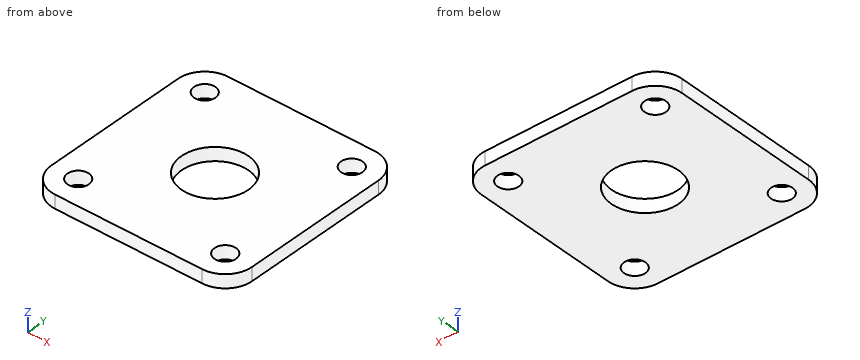
```python
from build123d import *

# Parameters (mm, degrees)
CYLINDER057_R       = 5
CYLINDER057_DEPTH   = 15
CYLINDER058_R       = 1.6
CYLINDER058_DEPTH   = 20
ARRAY001029_X_COUNT = 2
ARRAY001029_X_PITCH = 22
ARRAY001029_Y_COUNT = 2
ARRAY001029_Y_PITCH = 22
BOX007_W            = 30
BOX007_H            = 30
BOX007_DEPTH        = 2
FILLET013_R         = 4


with BuildPart() as side_bearing_central_hole_cylinder001:
    # Cylinder057 → Cylinder057 (new body)
    with BuildSketch(Plane(origin=(15, 15, -4), x_dir=(1, 0, 0), z_dir=(0, 0, 1))):
        Circle(CYLINDER057_R)
    extrude(amount=CYLINDER057_DEPTH)


with BuildPart() as fusion039:
    # Cylinder058 → Cylinder058 (new body)
    with BuildSketch(Plane(origin=(4, 4, -7), x_dir=(1, 0, 0), z_dir=(0, 0, 1))):
        Circle(CYLINDER058_R)
    extrude(amount=CYLINDER058_DEPTH)

    # Array001029 X: Fusion039 ×2


with BuildPart() as fusion039_1:
    add(fusion039.part)
    with Locations(*[(i * ARRAY001029_X_PITCH, 0, 0) for i in range(1, ARRAY001029_X_COUNT)]):
        add(fusion039.part)

    # Array001029 Y: Fusion039 ×2


with BuildPart() as fusion039_2:
    add(fusion039_1.part)
    with Locations(*[(0, i * ARRAY001029_Y_PITCH, 0) for i in range(1, ARRAY001029_Y_COUNT)]):
        add(fusion039_1.part)

    # Fusion039: union side bearing central hole cylinder001
    add(side_bearing_central_hole_cylinder001.part)


with BuildPart() as bearing_cover_fillet:
    # Box007 → Box007 (new body)
    with BuildSketch(Plane.XY):
        with Locations((15, 15)):
            Rectangle(BOX007_W, BOX007_H)
    extrude(amount=BOX007_DEPTH)

    # Cut023004: cut Fusion039
    add(fusion039_2.part, mode=Mode.SUBTRACT)

    # Fillet013
    fillet013_edges = [bearing_cover_fillet.edges().sort_by_distance(p)[0] for p in [
        (0, 0, 1),
        (0, 30, 1),
        (30, 0, 1),
        (30, 30, 1),
    ]]
    fillet(fillet013_edges, radius=FILLET013_R)


solid = bearing_cover_fillet.part
```
Part model, mm, in its own coordinate system. Give positions to 0.01 mm unless a question says otherwise; leave off trailing zeros. Order: outer loops, then holes, each group sorted by start corner. A loop starts at its lowest first (then second) coordinate and runs counter-clockwise, first axis right, second up. Notation, with made-up numbers: (82, -14) - (106, -14) arc R25 cw to (106, 24) - close; hole circle Ø10 at (16, 67). An arc over 180 degrees is marked (long way). Use one line per item in the form item = value.
Item 1: Probe probe 1 along X at (y, z) = (4, 0.75); probe 2 along Y at (x, z) = (26.75, 1.85). List the from-to ranges inside material, lowest first. Write a range as from..to.
Solution:
probe_1 = 0..2.4, 5.6..24.4, 27.6..30
probe_2 = 0.07..2.59, 5.41..24.59, 27.41..29.93
Item 2: Slice it at D-D on y = 3. Give the cut face in (x, z), and give its area (3 significant figures).
Solution:
outline = (0.13, 0) - (2.75, 0) - (2.75, 2) - (0.13, 2) - close; (5.25, 0) - (24.75, 0) - (24.75, 2) - (5.25, 2) - close; (27.25, 0) - (29.87, 0) - (29.87, 2) - (27.25, 2) - close
area = 49.5 mm2
Item 3: Slice it at C-C on z = 0.75. Give the cut face in (x, y), and give its area (3 significant figures).
Solution:
outline = (0, 4) arc R4 ccw to (4, 0) - (26, 0) arc R4 ccw to (30, 4) - (30, 26) arc R4 ccw to (26, 30) - (4, 30) arc R4 ccw to (0, 26) - close; hole circle Ø3.2 at (4, 4); hole circle Ø3.2 at (4, 26); hole circle Ø10 at (15, 15); hole circle Ø3.2 at (26, 4); hole circle Ø3.2 at (26, 26)
area = 776 mm2
Item 4: Slice it at B-B on x = 15. Give the cut face in (y, z), and give its area (3 significant figures).
Solution:
outline = (0, 0) - (10, 0) - (10, 2) - (0, 2) - close; (20, 0) - (30, 0) - (30, 2) - (20, 2) - close
area = 40.0 mm2
Item 5: Slice it at A-A on y = 11. Give the cut face in (x, z), and give its area (3 significant figures).
Solution:
outline = (0, 0) - (12, 0) - (12, 2) - (0, 2) - close; (18, 0) - (30, 0) - (30, 2) - (18, 2) - close
area = 48.0 mm2
